from build123d import *

# Parameters (mm, degrees)
SKETCH1_W           = 242.8875
SKETCH1_H           = 338.1375
SKETCH1_R           = 115.09375
BOSS_EXTRUDE1_DEPTH = 6.35
SKETCH7_R           = 1.905
CUT_EXTRUDE1_DEPTH  = 518.94193961


with BuildPart() as part:
    # Sketch1 → Boss-Extrude1 (new body)
    with BuildSketch(Plane(origin=(0, 0, 0), x_dir=(1, 0, 0), z_dir=(0, 1, 0))):
        with Locations((235.940705356, 205.764388046)):
            Rectangle(SKETCH1_W, SKETCH1_H)
        with Locations(Location((235.940705356, 158.139388046, 0), (0, 0, 270))):
            Circle(SKETCH1_R, mode=Mode.SUBTRACT)
    extrude(amount=BOSS_EXTRUDE1_DEPTH)

    # Sketch7 → Cut-Extrude1 (cut, through all)
    with BuildSketch(Plane.XZ):
        with Locations(Location((138.526478951, -44.416114451, 0), (0, 0, 270))):
            Circle(SKETCH7_R)
        with Locations(Location((128.389000388, -54.553593014, 0), (0, 0, 270))):
            Circle(SKETCH7_R)
        with Locations(Location((343.492410323, -54.553593014, 0), (0, 0, 90))):
            Circle(SKETCH7_R)
        with Locations(Location((333.354931761, -44.416114451, 0), (0, 0, 90))):
            Circle(SKETCH7_R)
        with Locations(Location((333.354931761, -271.862661641, 0), (0, 0, 270))):
            Circle(SKETCH7_R)
        with Locations(Location((343.492410323, -261.725183078, 0), (0, 0, 270))):
            Circle(SKETCH7_R)
        with Locations(Location((128.389000388, -261.725183078, 0), (0, 0, 90))):
            Circle(SKETCH7_R)
        with Locations(Location((138.526478951, -271.862661641, 0), (0, 0, 90))):
            Circle(SKETCH7_R)
    extrude(amount=-CUT_EXTRUDE1_DEPTH, mode=Mode.SUBTRACT)


solid = part.part
The listing builds one solid part. Answer for the finished solid, in the listing's coordinates (mm). Round coordinates to 2 decimals unless told otherwise and drop trailing zeros. Order: outer loops, then holes, each group sorted by start corner. A loop starts at its lowest first (then second) coordinate and runs counter-clockwise, first axis right, second up. Notation, with made-up numbers: (-26, 18.25) - (5, 18.25) arc R22 ccw to (5, 42.25) - close; hole circle Ø8 at (13.25, 30.25). An arc over 180 degrees is marked (long way). Write item = value, one per line. Start each with the question number.
1) Straight lines are drawn through the part: L1, parallel to X at y = 4, z = -160.5; L2, parallel to Z at x = 239.5, y = 5; L3, parallel to Z at x = 151, y = 2. For each, find the intervals that lie inside material, in ascending order.
2) For a pull along Z with two mould halves and no side action, classify faces 1 (the flat face through (234, 0, -283)), 2 (the flat face through (234, 3, -374.833)), 3 (the cylindrical face through (165.908, 3.131, -249.474)) as released by +Z, released by -Z, zero draft, split by the parting line, or undercut.
3) Section C-C, the plane y = 1.5 is taken. Count the separate pieces of the cut face and the enclosed holes in it, plus the area to 3 significant figures.
4) Section A-A, the plane x = 284 is taken. Write down the section's boundary in (y, z).
5) Section B-B, the plane z = -173 is taken. Write down the section's boundary in (x, y).
Results list:
q1.L1 = 114.5 to 120.87, 351.01 to 357.38
q1.L2 = -374.83 to -273.18, -43.1 to -36.7
q1.L3 = -374.83 to -235.8, -80.48 to -36.7
q2.face_1 = zero draft
q2.face_2 = released by -Z
q2.face_3 = undercut
q3.separate_pieces = 1
q3.enclosed_holes = 9
q3.area = 40,400 mm^2
q4.outline = (0, -374.83) - (6.35, -374.83) - (6.35, -262.72) - (0, -262.72) - close; (0, -53.56) - (6.35, -53.56) - (6.35, -36.7) - (0, -36.7) - close
q5.outline = (114.5, 0) - (121.81, 0) - (121.81, 6.35) - (114.5, 6.35) - close; (350.07, 0) - (357.38, 0) - (357.38, 6.35) - (350.07, 6.35) - close
